Work out the finished part from the listing and answer in its coordinate system (mm). Face numbers are marked on the shaded views. A direction names the side the tool comes from. Give positions to 0.01 mm unless a question says otherwise; leave off trailing zeros. Loops run counter-clockwise (first coordinate to the right, second up) from the corner with the lowest first, then second, coordinate; pieces in that order, holes last.
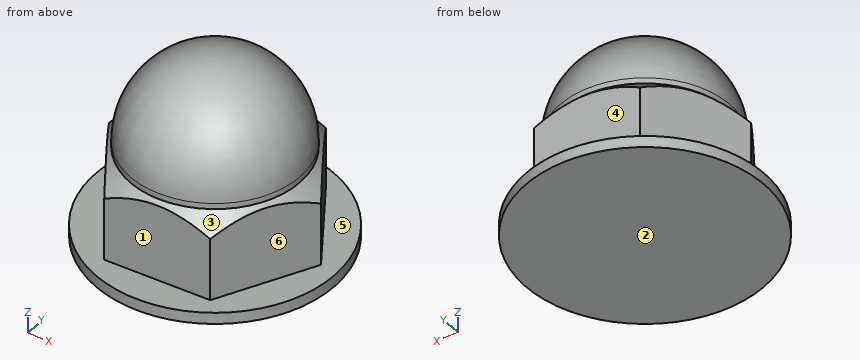
from build123d import *

# Parameters (mm, degrees)
SKETCH2_R           = 20.831287801
BOSS_EXTRUDE1_DEPTH = 2
BOSS_EXTRUDE2_DEPTH = 14
SKETCH4_R           = 20.916131801
SKETCH4_R_2         = 14.810913562
CUT_EXTRUDE1_DEPTH  = 14
CUT_EXTRUDE1_DRAFT  = -45
SKETCH5_R           = 14.810913562
BOSS_EXTRUDE3_DEPTH = 1
DOME1_FACE_RADIUS   = 14.810913562
DOME1_HEIGHT        = 15


with BuildPart() as part:
    # Sketch2 → Boss-Extrude1 (new body)
    with BuildSketch(Plane.XY):
        with Locations((74.414862174, 117.331579563)):
            Circle(SKETCH2_R)
    extrude(amount=BOSS_EXTRUDE1_DEPTH)

    # Sketch3 → Boss-Extrude2 (add)
    with BuildSketch(Plane.XY.offset(2)):
        Polygon((82.644465075, 133.181309802), (64.803394594, 132.383489858), (56.573791693, 116.533759619), (66.185259272, 101.481849324), (84.026329753, 102.279669268), (92.255932654, 118.129399507), align=None)
    extrude(amount=BOSS_EXTRUDE2_DEPTH)


with BuildPart() as cut_extrude1_tool:
    # Sketch4 → Cut-Extrude1 (with draft: the straight prism first)
    with BuildSketch(Plane.XY.offset(16)):
        with Locations((74.414862174, 117.331579563)):
            Circle(SKETCH4_R)
        with Locations((74.414862174, 117.331579563)):
            Circle(SKETCH4_R_2, mode=Mode.SUBTRACT)
    extrude(amount=-CUT_EXTRUDE1_DEPTH)
    # Cut-Extrude1: the draft: its side faces are tilted about the plane it starts from
    cut_extrude1_sides = [cut_extrude1_tool.faces().sort_by_distance(p)[0] for p in [
        (53.498730373, 117.331579563, 9),
        (59.603948612, 117.331579563, 9),
    ]]
    draft(cut_extrude1_sides, Plane.XY.offset(16), CUT_EXTRUDE1_DRAFT)


with BuildPart() as part_1:
    add(part.part)

    # Cut-Extrude1: cut by cut_extrude1_tool
    add(cut_extrude1_tool.part, mode=Mode.SUBTRACT)

    # Sketch5 → Boss-Extrude3 (add)
    with BuildSketch(Plane.XY.offset(16)):
        with Locations((74.414862174, 117.331579563)):
            Circle(SKETCH5_R)
    extrude(amount=BOSS_EXTRUDE3_DEPTH)

    # Dome1: an elliptical dome of height H over a round flat face of radius A is half a spheroid: the quarter ellipse of half axes A and H revolved about the face's axis
    with BuildSketch(Plane((74.414862174, 117.331579563, 17), x_dir=(0, 1, 0), z_dir=(1, 0, 0)), mode=Mode.PRIVATE) as dome1_quarter:
        Ellipse(DOME1_FACE_RADIUS, DOME1_HEIGHT)
        Rectangle(DOME1_FACE_RADIUS, DOME1_HEIGHT, align=(Align.MIN, Align.MIN), mode=Mode.INTERSECT)
    revolve(dome1_quarter.sketch, axis=Axis((74.414862174, 117.331579563, 17), (0, 0, 1)))


solid = part_1.part
Item 1: Flat-ended cylindrical pins translate along their axes: pin 1 Ø3 at (y, z) = (115, 26.5) entering from -X; pin 2 Ø4 at (x, z) = (60, 8) entering from -Y; pin 3 Ø3 at (y, z) = (106.5, 7.5) entering from +X. Find the tip coordinate at first contact, or state that the pin passes through.
Item 2: Determine the mould class of the marked faces 1, 2 and 3 for opening direction Z: released by +Z, released by -Z, zero draft, split by the parting line, or undercut.
Item 3: Find section A-A, the plane z = 5.5. Write down the section's boundary in (x, y), plus the area to 3 significant figures.
Item 4: For the marked faces 4, 5 and 6, determine the directions among +Z, -Z, +X, -X, +Y, -Y from which every point of the face is accessible in a straight line to the end or side of a thin tool.
Item 5: Consider line 1 (Z direction, x = 63.5, y = 104); line 2 (X direction, y = 117, z = 16); line 3 (Y direction, x = 62, z = 19.5). Determine where each line is inside the solid, lowest interval first.
Ans:
1. pin 1: stops at x = 62.07
1. pin 2: stops at y = 108.04
1. pin 3: stops at x = 87
2. face 1: zero draft
2. face 2: released by -Z
2. face 3: released by +Z
3. outline: (56.57, 116.53) - (66.19, 101.48) - (84.03, 102.28) - (92.26, 118.13) - (82.64, 133.18) - (64.8, 132.38) - close
3. area: 829 mm2
4. face 4: +Z, -X, +Y
4. face 5: +Z
4. face 6: +Z, +X, -Y
5. line 1: z = 0 to 2
5. line 2: x = 59.61 to 89.22
5. line 3: y = 109.64 to 125.02
